Here's how the part is built. I have some questions about the finished solid (model axes, mm). Face numbers are marked on the shaded views. A direction names the side the tool comes from. Round coordinates to 2 decimals unless told otherwise and drop trailing zeros. Loops run counter-clockwise (first coordinate to the right, second up) from the corner with the lowest first, then second, coordinate; pieces in that order, holes last. Notation, with made-up numbers: (9.25, 60) - (45.25, 60) arc R22 ccw to (45.25, 85) - close; hole circle Ø6 at (-11, 4). An arc over 180 degrees is marked (long way). Return JSON: item names as keys, results as strings. Group by question number.
```python
from build123d import *

# Parameters (mm, degrees)
F1_DEPTH = 5
F3_DEPTH = 25
F5_W     = 13.2
F5_H     = 14.5
F5_W_2   = 42
F5_H_2   = 21
F6_DEPTH = 5


with BuildPart() as f1:
    # F0 (on Top) → F1 (new body)
    with BuildSketch(Plane.XY):
        Polygon((68.193161, 51.273486), (-46.306839, 51.273486), (-46.306839, -61.726514), (-21.806839, -84.226514), (43.693161, -84.226514), (68.193161, -61.726514), align=None)
    extrude(amount=F1_DEPTH)

    # F2 (on face) → F3 (join)
    with BuildSketch(Plane.XY.offset(5)):
        Polygon((68.193161, -61.726514), (68.193161, 51.273486), (-46.306839, 51.273486), (-46.306839, -61.726514), (-21.806839, -84.226514), (43.693161, -84.226514), align=None)
        Polygon((-19.859262, -79.226514), (-41.306839, -59.52976), (-41.306839, 46.273486), (63.193161, 46.273486), (63.193161, -59.52976), (41.745585, -79.226514), align=None, mode=Mode.SUBTRACT)
    extrude(amount=F3_DEPTH)

    # F5 (on face) → F6 (cut, through all)
    with BuildSketch(Plane.YZ.offset(68.193161)):
        with Locations((-20.926514, 18.75)):
            Rectangle(F5_W, F5_H)
        with Locations((22.673486, 15.5)):
            Rectangle(F5_W_2, F5_H_2)
    extrude(amount=-F6_DEPTH, mode=Mode.SUBTRACT)


solid = f1.part
```
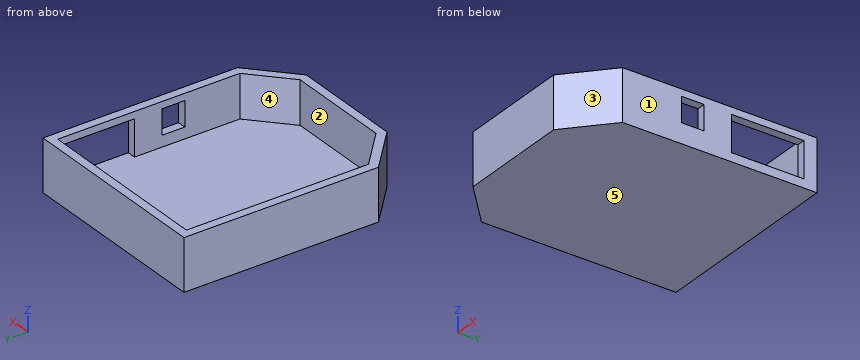
Q1. Please list where these lines run through material, in increasing order: line 1 (Y direction, x = -17.5, z = 20.25); line 2 (X direction, y = -48, z = 25.75); line 3 (X direction, y = 26, z = 19).
Q2. Imagine slicing it at B-B, the plane z = 15.75. List the corners of the cut face in (x, y) for me.
Q3. For the marked faces 1 and 2, which set-ups out of +Z, -Z, +X, -X, +Y, -Y let a thin tool reach every point of the face, with its end or its side?
Q4. Will these pins go through, and if not, where does the flat tip stop? pin 1 Ø5.5 at (x, z) = (66.5, 18.5) entering from -Y; pin 2 Ø1.5 at (y, z) = (18.5, 11) entering from +X; pin 3 Ø6 at (x, y) = (-21, 5.5) entering from +Z.
Q5. If we mould it in two halves opening along X, with no side actions, what happens to the marked faces 3, 4 and 5? For each: +X half, -X half, draft (parallel to the pull), parting line (faces both ways), or undercut.
Q6. Imagine slicing it at A-A, the plane y = 29.5. List the corners of the cut face in (x, z) for me.
Q7. Imagine slicing it at D-D, the plane x = -15.5. List the corners of the cut face in (y, z) for me, and give its area (4 significant figures).
Q8. Imagine slicing it at C-C, the plane y = -43.5. List the corners of the cut face in (x, z) for me.
Output values:
{
 "1": {"line 1": "y = -84.23 to -79.23, 46.27 to 51.27", "line 2": "x = -46.31 to -41.31, 63.19 to 68.19", "line 3": "x = -46.31 to -41.31"},
 "2": {"outline": "(-46.31, -61.73) - (-21.81, -84.23) - (43.69, -84.23) - (68.19, -61.73) - (68.19, -27.53) - (63.19, -27.53) - (63.19, -59.53) - (41.75, -79.23) - (-19.86, -79.23) - (-41.31, -59.53) - (-41.31, 46.27) - (63.19, 46.27) - (63.19, 43.67) - (68.19, 43.67) - (68.19, 51.27) - (-46.31, 51.27) - close; (63.19, -14.33) - (68.19, -14.33) - (68.19, 1.67) - (63.19, 1.67) - close"},
 "3": {"face 1": "+Z, -Z, +X, +Y, -Y", "face 2": "+Z"},
 "4": {"pin 1": "stops at y = -65.81", "pin 2": "stops at x = -41.31", "pin 3": "stops at z = 5"},
 "5": {"face 3": "+X half", "face 4": "undercut", "face 5": "draft"},
 "6": {"outline": "(-46.31, 0) - (68.19, 0) - (68.19, 5) - (-41.31, 5) - (-41.31, 30) - (-46.31, 30) - close; (63.19, 26) - (68.19, 26) - (68.19, 30) - (63.19, 30) - close"},
 "7": {"outline": "(-84.23, 0) - (51.27, 0) - (51.27, 30) - (46.27, 30) - (46.27, 5) - (-79.23, 5) - (-79.23, 30) - (-84.23, 30) - close", "area": "927.5 mm^2"},
 "8": {"outline": "(-46.31, 0) - (68.19, 0) - (68.19, 30) - (63.19, 30) - (63.19, 5) - (-41.31, 5) - (-41.31, 30) - (-46.31, 30) - close"}
}
